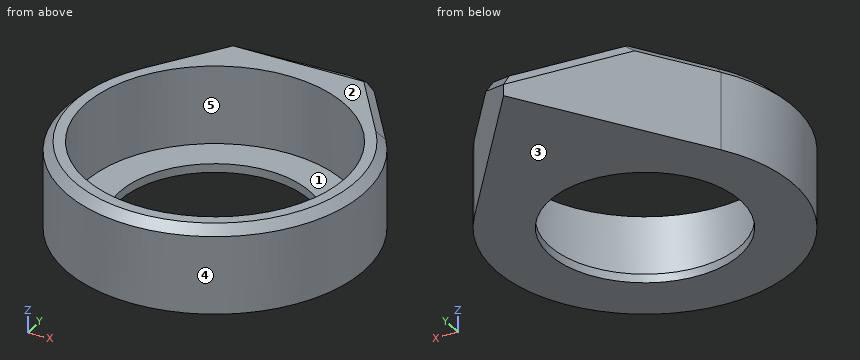
```python
from build123d import *

# Parameters (mm, degrees)
F0_R         = 14.75
F0_R_2       = 11
F1_DEPTH     = 0.5
F3_DEPTH     = 10
F4_R         = 15
F5_DEPTH     = 9
F8_DEPTH     = 12.5
F9_T1_DEPTH  = 11.9079151816
F9_T3_DEPTH  = 20.7352111954
F9_T5_DEPTH  = 20.7352111954
F9_T7_DEPTH  = 11.9079151816
F9_T10_ANGLE = 250.6333606171
F6_R         = 11
F10_DEPTH    = 25


# Not quite as in the source:
# - a fillet or chamfer that OpenCascade refuses, or shapes differently, is made with other operations: its cross-section is extruded or revolved along the edge and cut away or added


with BuildPart() as f1:
    # F0 (on Top) → F1 (new body)
    with BuildSketch(Plane.XY):
        Circle(F0_R)
        Circle(F0_R_2, mode=Mode.SUBTRACT)
    extrude(amount=F1_DEPTH)

    # F2 (on Top) → F3 (join)
    with BuildSketch(Plane.XY):
        with BuildLine():
            Line((0, 29.8393759876), (-14.0754708725, 9.972142183))
            ThreePointArc((-14.0754708725, 9.972142183), (0, -17.25), (14.0754708725, 9.972142183))
            Line((14.0754708725, 9.972142183), (0, 29.8393759876))
        make_face()
    extrude(amount=F3_DEPTH)

    # F4 (on face) → F5 (cut)
    with BuildSketch(Plane.XY.offset(10)):
        Circle(F4_R)
    extrude(amount=-F5_DEPTH, mode=Mode.SUBTRACT)

    # F7 (on Right) → F8 (cut, symmetric)
    with BuildSketch(Plane.YZ):
        Polygon((30.5235402449, 1.681677395), (30.5303540081, 10.6816748157), (16.5303540081, 10.6816748157), align=None)
    extrude(amount=F8_DEPTH, both=True, mode=Mode.SUBTRACT)

    # F9: chamfer of 1 on 5 edges, made by hand

    # F9_s2 → F9_t1 (cut)
    with BuildSketch(Plane(origin=(0, 0, 0), x_dir=(0, 0, 1), z_dir=(-0.578095199, 0.8159693259, 0))):
        Polygon((9, 17.25), (10, 16.25), (10, 17.25), align=None)
    extrude(amount=F9_T1_DEPTH, mode=Mode.SUBTRACT)

    # F9_s4 → F9_t3 (cut)
    with BuildSketch(Plane(origin=(-11.4991327342, 16.2307862132, -10.4391545701), x_dir=(0.8159693259, 0.578095199, 0), z_dir=(0.5118849348, -0.7225149178, 0.4646999108))):
        Polygon((17.25, 12.4696557739), (16.5627169892, 13.4195021219), (17.25, 13.1932286048), align=None)
    extrude(amount=F9_T3_DEPTH, mode=Mode.SUBTRACT)

    # F9_s6 → F9_t5 (cut)
    with BuildSketch(Plane(origin=(0.8850905039, 1.2492868011, -0.8035037766), x_dir=(-0.8159693259, 0.578095199, 0), z_dir=(0.5118849348, 0.7225149178, -0.4646999108))):
        Polygon((17.25, 12.4696557739), (16.5627169892, 13.4195021219), (17.25, 13.1932286048), align=None)
    extrude(amount=F9_T5_DEPTH, mode=Mode.SUBTRACT)

    # F9_s8 → F9_t7 (cut)
    with BuildSketch(Plane(origin=(6.8839085967, 9.7164935241, 0), x_dir=(0, 0, 1), z_dir=(-0.578095199, -0.8159693259, 0))):
        Polygon((9, 17.25), (10, 16.25), (10, 17.25), align=None)
    extrude(amount=F9_T7_DEPTH, mode=Mode.SUBTRACT)

    # F9_s9 → F9_t10 (revolve, cut)
    with BuildSketch(Plane(origin=(0, 0, 0), x_dir=(0, 0, 1), z_dir=(0.578095199, 0.8159693259, 0))):
        Polygon((10, -16.25), (9, -17.25), (10, -17.25), align=None)
    revolve(axis=Axis((0, 0, 10), (0, 0, 1)), revolution_arc=F9_T10_ANGLE, mode=Mode.SUBTRACT)

    # F6 (on face) → F10 (cut)
    with BuildSketch(Plane.XY.offset(1)):
        Circle(F6_R)
    extrude(amount=-F10_DEPTH, mode=Mode.SUBTRACT)


solid = f1.part
```
Model file for the job. Use its own axes, mm. Face numbers are marked on the shaded views. A direction names the side the tool comes from. Round coordinates to 2 decimals unless told otherwise and drop trailing zeros. Write each loop counter-clockwise with the first axis right and the second up, starting at its lowest first coordinate (ties: lowest second). Pieces come first, ordered by that corner, then holes. Notation, with made-up numbers: (-37, 57) - (-14, 57) arc R18 ccw to (-14, 85) - close; hole circle Ø11 at (84, 65). An arc over 180 degrees is marked (long way). Use CSV: the item, a comma, the result in double quotes. Start each with the question number.
Item 1: Band-saw the part on B-B (z = 3.75). Write the cut outline in (x, y), and give its area (3 significant figures).
Item 2: Band-saw the part on A-A (y = 0). Write the cut outline in (x, z), and give its area (3 significant figures).
Item 3: Two-plate mould, pull along Y, no slides. Class the marked faces 3, 4 and 5: released by +Y, released by -Y, zero draft, split by the parting line, or undercut.
Item 4: Band-saw the part on D-D (y = 22.5). Write the cut outline in (x, z).
Item 5: Drill centre lines: L1, parallel to X at y = -0.5, z = 1.5; L2, parallel to Y at x = 2, z = 3.5; L3, parallel to Y at x = 12, z = 7.75. Where is each one in solid material? Low to high. Write a range as [from, to].
Item 6: Tool access for the marked faces 1 and 2: list every direction of +Z, -Z, +X, -X, +Y, -Y with a clear straight run to the whole face (end or side of a thin tool).
Item 7: Band-saw the part on C-C (z = 6.75). Write the cut outline in (x, y).
Item 8: Pin check, flat tips, straight feed: P1, Ø1.5, axis at y = 1.5, z = 9, coming from the -X side; P2, Ø3, axis at x = -9.5, y = -7.5, coming from the +Z side; P3, Ø1.5, axis at y = 6, z = 8.5, coming from the +X side. Stop position of each tip, or through.
Checked values:
1,outline,"(-14.08, 9.97) arc R17.25 ccw (long way) to (14.08, 9.97) - (2.69, 26.04) - (0.95, 27.31) - (-0.95, 27.31) - (-2.69, 26.04) - close; hole circle Ø30 at (0, 0)"
1,area,"358 mm²"
2,outline,"(-17.25, 0) - (-11, 0) - (-11, 1) - (-15, 1) - (-15, 10) - (-16.25, 10) - (-17.25, 9) - close; (11, 0) - (17.25, 0) - (17.25, 9) - (16.25, 10) - (15, 10) - (15, 1) - (11, 1) - close"
2,area,"52.0 mm²"
3,face 3,"zero draft"
3,face 4,"split by the parting line"
3,face 5,"undercut"
4,outline,"(-5.2, 0) - (5.2, 0) - (5.2, 6.03) - (4.36, 6.84) - (-4.36, 6.84) - (-5.2, 6.03) - close"
5,L1,"x = [-17.24, -14.99], [14.99, 17.24]"
5,L2,"y = [-17.13, -14.87], [14.87, 26.73]"
5,L3,"y = [-12.39, -9], [9, 12.9]"
6,face 1,"+Z"
6,face 2,"+Z, +X, -X, +Y, -Y"
7,outline,"(-14.08, 9.97) arc R17.25 ccw (long way) to (14.08, 9.97) - (6, 21.37) - (4.26, 22.64) - (-4.26, 22.64) - (-6, 21.37) - close; hole circle Ø30 at (0, 0)"
8,P1,"stops at x = -17.23"
8,P2,"stops at z = 1"
8,P3,"stops at x = 16.43"
